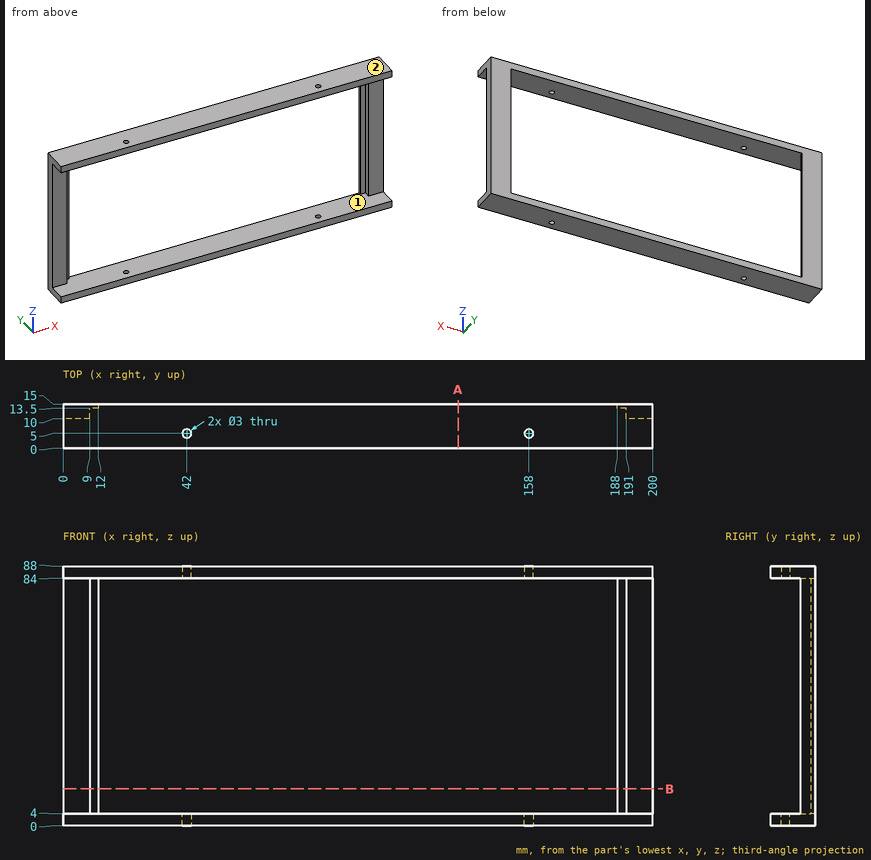
Geometry check sheet. Reference: drawing and pictorial views, mm from the part's lowest x, y, z. Coordinates: 2 decimals unless noted, no trailing zeros. Write each loop counter-clockwise with the first axis right and the second up, starting at its lowest first coordinate (ties: lowest second). Pieces come first, ordered by that corner, then holes. Notation, with made-up numbers: M 57.5,-26.5 L 64.5,-26.5 A11 ccw 64.5,-5.5 Z; hole C 70.5,29 d8. An arc over 180 degrees is marked long. Write item = value, one per line. Start each with the question number.
1. Sectioned sample at B-B (z = 12.5). Record the cut outline in (x, y).
2. Go/stop test with flat-tipped pins: pin 1 (3.5 mm diameter, centred on x = 158, y = 5, fed in from +Z); pin 2 (3 mm diameter, centred on y = 8, z = 75.5, fed in from -X); pin 3 (2.5 mm diameter, centred on x = 190, z = 34.5, fed in from -Y). Record where each tip stops, or that it passes through.
3. Thickness scan on probe 1 along Z at (x, y) = (90, 8.75); probe 2 along X at (y, z) = (13.75, 14.5); probe 3 along Y at (x, z) = (42, 85.1). Record the ranges inside material, lowest first.
4. Sectioned sample at A-A (x = 134). Record the cut outline in (y, z), then the cut area to 3 significant figures.
5. Mould release check, pull along X, two halves, no side actions. Record for the marked faces 1 and 2: pulls with the +X half, pulls with the -X half, needs draft (parallel to the pull), parting line crosses it, or undercut.
The answers:
q1.outline = M 0,10 L 9,10 L 9,13.5 L 12,13.5 L 12,15 L 0,15 Z; M 188,13.5 L 191,13.5 L 191,10 L 200,10 L 200,15 L 188,15 Z
q2.pin_1 = 88
q2.pin_2 = through
q2.pin_3 = 10
q3.probe_1 = 0 to 4, 84 to 88
q3.probe_2 = 0 to 12, 188 to 200
q3.probe_3 = 0 to 3.5, 6.5 to 15
q4.outline = M 0,0 L 15,0 L 15,4 L 0,4 Z; M 0,84 L 15,84 L 15,88 L 0,88 Z
q4.area = 120 mm²
q5.face_1 = undercut
q5.face_2 = needs draft
